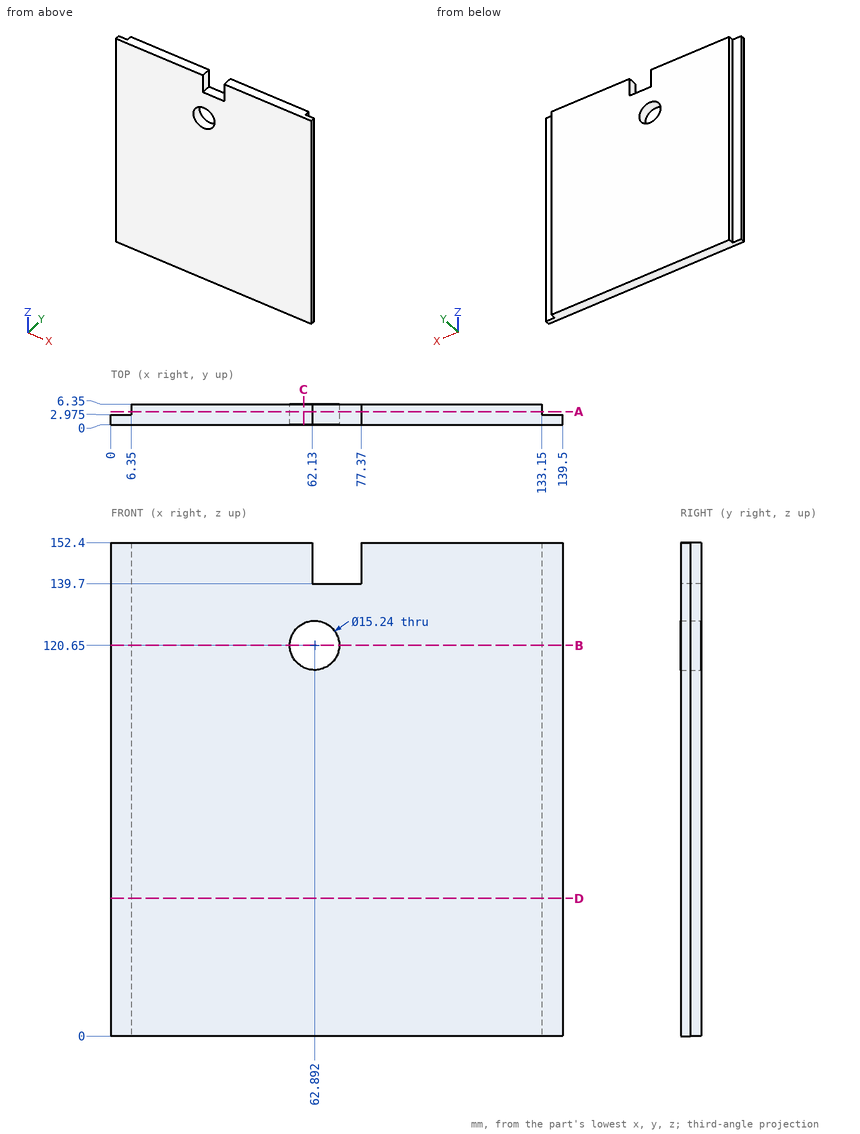
Study the drawing (mm; zero at the part's minimum x, y, z) and answer. Round coordinates to 2 decimals unless told otherwise and drop trailing zeros. Loops run counter-clockwise (first coordinate to the right, second up) from the corner with the lowest first, then second, coordinate; pieces in that order, holes last. Notation, with made-up numbers: (5.25, 82.25) -> (27.25, 82.25) arc R16 cw to (27.25, 107.25) -> close; hole circle Ø1 at (-34.5, 31.25). An arc over 180 degrees is marked (long way). One line per item, written item: value.
1) Consider L1, parallel to X at y = 4.75, z = 120.65; L2, parallel to X at y = 2.5, z = 142.5; L3, parallel to X at y = 5, z = 87. Determine where each line is inside the solid, lowest interval first. Write a range as [from, to].
Answer list:
L1: x = [6.35, 55.27], [70.51, 133.15]
L2: x = [0, 62.13], [77.37, 139.5]
L3: x = [6.35, 133.15]
2) A cutting plane is placed at A-A (y = 4). Determine the outline of the cut face in (x, z).
Answer list:
outline: (6.35, 0) -> (133.15, 0) -> (133.15, 152.4) -> (77.37, 152.4) -> (77.37, 139.7) -> (62.13, 139.7) -> (62.13, 152.4) -> (6.35, 152.4) -> close; hole circle Ø15.24 at (62.89, 120.65)
3) A cutting plane is placed at D-D (z = 42.5). Determine the outline of the cut face in (x, y) (3 decimals).
Answer list:
outline: (0, 0) -> (139.5, 0) -> (139.5, 2.975) -> (133.15, 2.975) -> (133.15, 6.35) -> (6.35, 6.35) -> (6.35, 2.975) -> (0, 2.975) -> close
4) A cutting plane is placed at C-C (x = 59.5). Determine the outline of the cut face in (y, z).
Answer list:
outline: (0, 0) -> (6.35, 0) -> (6.35, 113.83) -> (0, 113.83) -> close; (0, 127.47) -> (6.35, 127.47) -> (6.35, 152.4) -> (0, 152.4) -> close
5) Flat-ended cylindrical pins translate along their axes: P1, Ø1, axis at x = 63.5, y = 1, coming from the +Z side; P2, Ø3.5, axis at y = 4.5, z = 51.5, coming from the -X side; P3, Ø3, axis at x = 135, z = 46, coming from the +Y side (3 decimals); P4, Ø1, axis at y = 5.5, z = 64.5, coming from the +X side. Find the tip coordinate at first contact, or state that the pin passes through.
Answer list:
P1: stops at z = 139.7
P2: stops at x = 0
P3: stops at y = 2.975
P4: stops at x = 133.15
6) A cutting plane is placed at B-B (z = 120.65). Determine the outline of the cut face in (x, y) (3 decimals).
Answer list:
outline: (0, 0) -> (55.272, 0) -> (55.272, 6.35) -> (6.35, 6.35) -> (6.35, 2.975) -> (0, 2.975) -> close; (70.512, 0) -> (139.5, 0) -> (139.5, 2.975) -> (133.15, 2.975) -> (133.15, 6.35) -> (70.512, 6.35) -> close
